Source: CAD feature listing. Evaluate the final solid. Frame: model axes, mm. A direction names the side the tool comes from. Round coordinates to 2 decimals unless told otherwise and drop trailing zeros. Write each loop counter-clockwise with the first axis right and the second up, starting at its lowest first coordinate (ties: lowest second). Pieces come first, ordered by that corner, then holes. Notation, with made-up numbers: M 57,62 L 96,62 A13 cw 96,67 Z; hole C 49.25,-36 d2. An arc over 180 degrees is marked long. Answer in a Markdown table with one row per item.
from build123d import *

# Parameters (mm, degrees)
F1_DEPTH = 2
F4_COUNT = 6
F4_ANGLE = 300


with BuildPart() as f1:
    # F0 (on Top) → F1 (new body)
    with BuildSketch(Plane.XY):
        Polygon((4.630033, 25.07996), (24.53151, 47.784701), (3.992958, 36.931831), (35.760634, 69.906734), (4.827321, 57.226207), (17.619738, 92.714362), (0, 70.044786), (0, 0), (3.223337, 0), (10.876871, 23.889082), align=None)
    extrude(amount=F1_DEPTH)

    # F2: F1 across plane


with BuildPart() as f1_1:
    add(f1.part)
    add(f1.part.mirror(Plane.YZ))

    # F4: F1 ×6 about axis
    f4_axis = Axis((0, 0, 4.113019), (0, 0, 1))


with BuildPart() as f1_2:
    add(f1_1.part)
    for i in range(1, F4_COUNT):
        add(f1_1.part.rotate(f4_axis, i * F4_ANGLE / (F4_COUNT - 1)))


solid = f1_2.part
Q1. Pull-direction query (X, two-part tool) for faces 1 (the flat face through (65.382, -14.065, 0.986)), 2 (the flat face through (-66.15, -48.51, 0.99)), 3 (the flat face through (20.511, -63.655, 0.986)); classes: pulls with the +X half, pulls with the -X half, needs draft (parallel to the pull), parting line crosses it, or undercut.
Solutions:
| item | result |
|---|---|
| face 1 | pulls with the +X half |
| face 2 | pulls with the -X half |
| face 3 | undercut |
Q2. Material intervals for probe 1 along X at (y, z) = (-63.5, 1.4); probe 2 along Y at (x, z) = (75.5, 1); probe 3 along Y at (x, z) = (-60, 0.95), sorted ascending.
Solutions:
| item | result |
|---|---|
| probe 1 | x = -42.99 to -41.96, -29.59 to -20.13, -7.09 to 7.09, 20.13 to 29.59, 41.96 to 42.99 |
| probe 2 | y = -32.97 to -28.66, -6.24 to -4.71, 4.71 to 6.24, 28.66 to 32.97 |
| probe 3 | y = -48.02 to -25.87, -18.23 to -8.55, 8.55 to 18.23, 25.87 to 48.02 |
Q3. Access query for faces 4 (the flat face through (-8.933, 81.538, 0.986)), 5 (the flat face through (-24.19, 30.64, 0.99)), 6 (the flat face through (66.15, 48.51, 0.99)). Directions: +Z, -Z, +X, -X, +Y, -Y. A direction counts if a zero-diameter tool reaches every point of the face in a straight line with its end or side. Return the directions, or none.
Solutions:
| item | result |
|---|---|
| face 4 | +Z, -Z, +Y |
| face 5 | +Z, -Z |
| face 6 | +Z, -Z, +X |
Q4. Section B-B (x = -68). Return loops of the section in (y, z), and give its area (3 significant figures).
Solutions:
| item | result |
|---|---|
| outline | M -57.49,0 L -53.06,0 L -53.06,2 L -57.49,2 Z; M -34.01,0 L -27.31,0 L -27.31,2 L -34.01,2 Z; M -12.04,0 L -6.57,0 L -6.57,2 L -12.04,2 Z; M 6.57,0 L 12.04,0 L 12.04,2 L 6.57,2 Z; M 27.31,0 L 34.01,0 L 34.01,2 L 27.31,2 Z; M 53.06,0 L 57.49,0 L 57.49,2 L 53.06,2 Z |
| area | 66.4 mm2 |
Q5. Section C-C (y = -53). Return loops of the section in (x, z).
Solutions:
| item | result |
|---|---|
| outline | M -67.98,0 L -64.21,0 L -64.21,2 L -67.98,2 Z; M -44.41,0 L -38.94,0 L -38.94,2 L -44.41,2 Z; M -19.47,0 L 19.47,0 L 19.47,2 L -19.47,2 Z; M 38.94,0 L 44.41,0 L 44.41,2 L 38.94,2 Z; M 64.21,0 L 67.98,0 L 67.98,2 L 64.21,2 Z |
Q6. Section A-A (y = 75.5). Return loops of the section in (x, z).
Solutions:
| item | result |
|---|---|
| outline | M -11.41,0 L -4.24,0 L -4.24,2 L -11.41,2 Z; M 4.24,0 L 11.41,0 L 11.41,2 L 4.24,2 Z |
